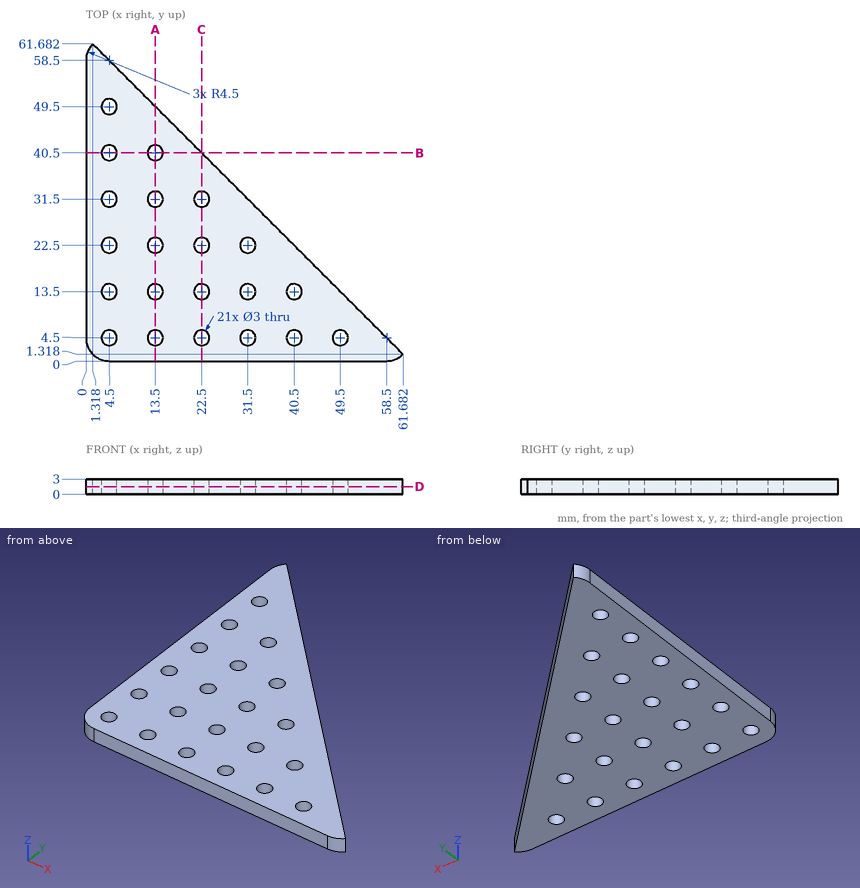
Source: three-view drawing plus pictorial views. Frame: mm from the lowest corner of the part. Coordinates: 2 decimals unless noted, no trailing zeros. Order: outer loops, then holes, each group sorted by start corner. A loop starts at its lowest first (then second) coordinate and runs counter-clockwise, first axis right, second up.
Item 1: Cut plane A-A (x = 13.5). Return loops of the section in (y, z).
Output values:
outline: (0, 0) - (3, 0) - (3, 3) - (0, 3) - close; (6, 0) - (12, 0) - (12, 3) - (6, 3) - close; (15, 0) - (21, 0) - (21, 3) - (15, 3) - close; (24, 0) - (30, 0) - (30, 3) - (24, 3) - close; (33, 0) - (39, 0) - (39, 3) - (33, 3) - close; (42, 0) - (49.5, 0) - (49.5, 3) - (42, 3) - close
Item 2: Cut plane D-D (z = 1.5). Count the separate pieces of the cut face and the enclosed holes in it, plus the area to 3 significant figures.
Output values:
separate pieces: 1
enclosed holes: 21
area: 1,830 mm2
Item 3: First-contact query: P1, Ø1.8, axis at x = 13.5, y = 31.5, coming from the -Z side; P2, Ø1, axis at x = 16, z = 1.5, coming from the +Y side; P3, Ø1, axis at y = 9, z = 2.5, coming from the +X side; P4, Ø1, axis at y = 51.5, z = 2, coming from the +X side. Flat tips, straight axial feed; report the tip coordinate or a pass-through.
Output values:
P1: passes through
P2: stops at y = 47.5
P3: stops at x = 54.5
P4: stops at x = 12
Item 4: Cut plane C-C (x = 22.5). Return loops of the section in (y, z).
Output values:
outline: (0, 0) - (3, 0) - (3, 3) - (0, 3) - close; (6, 0) - (12, 0) - (12, 3) - (6, 3) - close; (15, 0) - (21, 0) - (21, 3) - (15, 3) - close; (24, 0) - (30, 0) - (30, 3) - (24, 3) - close; (33, 0) - (40.5, 0) - (40.5, 3) - (33, 3) - close
Item 5: Cut plane B-B (y = 40.5). Return loops of the section in (x, z).
Output values:
outline: (0, 0) - (3, 0) - (3, 3) - (0, 3) - close; (6, 0) - (12, 0) - (12, 3) - (6, 3) - close; (15, 0) - (22.5, 0) - (22.5, 3) - (15, 3) - close
Item 6: Material intervals for line 1 (Y direction, x = 22.5, z = 1.05); line 2 (Y direction, x = 13.5, z = 2.25); line 3 (Y direction, x = 31.5, z = 1.5), sorted ascending.
Output values:
line 1: y = 0 to 3, 6 to 12, 15 to 21, 24 to 30, 33 to 40.5
line 2: y = 0 to 3, 6 to 12, 15 to 21, 24 to 30, 33 to 39, 42 to 49.5
line 3: y = 0 to 3, 6 to 12, 15 to 21, 24 to 31.5
